Input: dimensioned drawing with shaded views. Units: mm. Origin: part minimum x, y, z. Coordinates: 2 decimals unless noted, no trailing zeros. Order: outer loops, then holes, each group sorted by start corner. A loop starts at its lowest first (then second) coordinate and runs counter-clockwise, first axis right, second up.
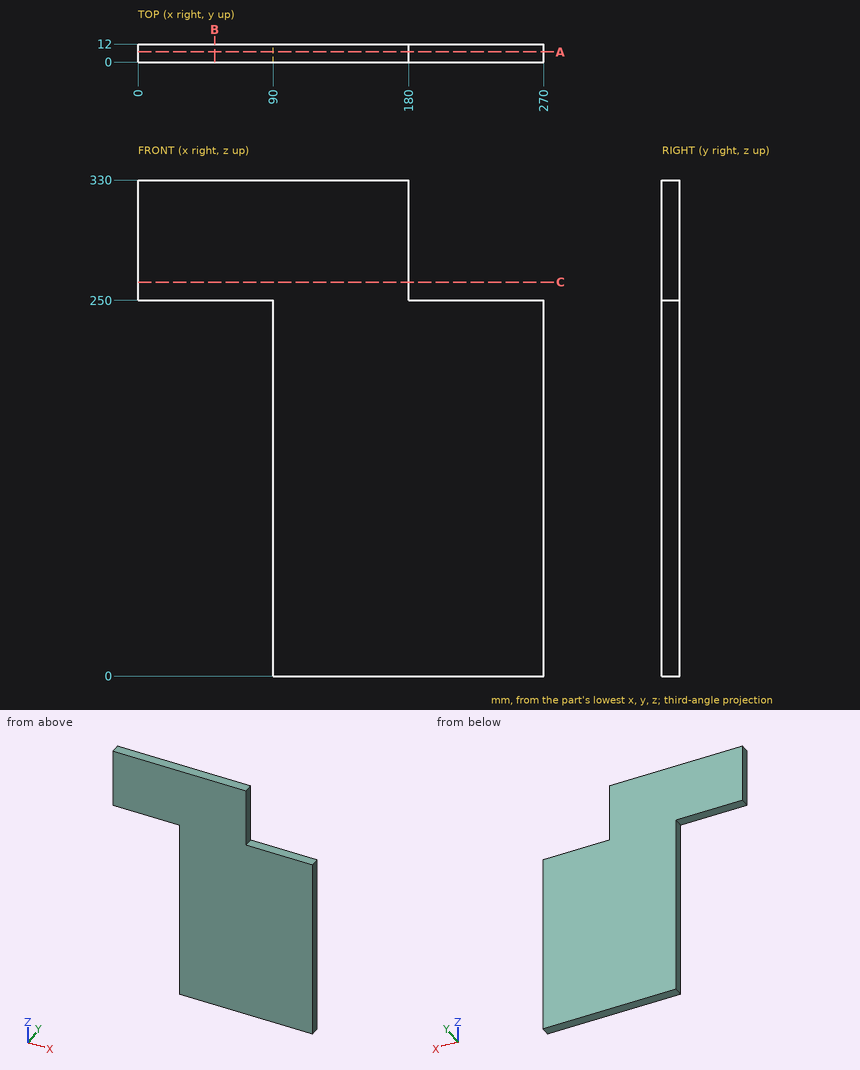
1. Section query B-B, the plane x = 51. Output: boundary loops of the cut face in (y, z), plus the area to 3 significant figures.
2. Material intervals for line 1 along X through (y, z) = (4, 32); line 2 along X through (y, z) = (5.75, 274.5); line 3 along Z through (x, y) = (192, 2.75), sorted ascending.
3. Section query C-C, the plane z = 262. Output: boundary loops of the cut face in (x, y), plus the area to 3 significant figures.
4. Contact query for flat-ended pins moving along their axis: P1, Ø6, axis at y = 7.5, z = 58.5, coming from the -X side; P2, Ø6, axis at x = 232, y = 5.5, coming from the +Z side; P3, Ø6, axis at y = 4.5, z = 270.5, coming from the +X side; P4, Ø1.5, axis at y = 10.5, z = 292, coming from the -X side. Output: stop coordinate, or through.
5. Section query A-A, the plane y = 6.75. Output: boundary loops of the cut face in (x, z), plus the area to 3 significant figures.
Answer key:
1. outline: (0, 250) - (12, 250) - (12, 330) - (0, 330) - close
1. area: 960 mm2
2. line 1: x = 90 to 270
2. line 2: x = 0 to 180
2. line 3: z = 0 to 250
3. outline: (0, 0) - (180, 0) - (180, 12) - (0, 12) - close
3. area: 2,160 mm2
4. P1: stops at x = 90
4. P2: stops at z = 250
4. P3: stops at x = 180
4. P4: stops at x = 0
5. outline: (0, 250) - (90, 250) - (90, 0) - (270, 0) - (270, 250) - (180, 250) - (180, 330) - (0, 330) - close
5. area: 59,400 mm2
